Autodesk Inventor part; units mm, degrees
ref_plane "YZ Plane" through (0, 0, 0) normal (1, 0, 0) x (0, 1, 0)
ref_plane "XZ Plane" through (0, 0, 0) normal (0, 1, 0) x (-1, 0, 0)
ref_plane "XY Plane" through (0, 0, 0) normal (0, 0, 1) x (1, 0, 0)
sketch "Sketch1" plane through (0, 0, 0) normal (0, 1, 0) x (-1, 0, 0)
  circle A0 centre (0, 0) radius 17.5
  dimension "d0" = 35
extrude "Base" add sketch "Sketch1" along normal blind 10
sketch "Sketch2" plane through (0, 10, 0) normal (0, 1, 0) x (1, 0, 0)
  circle A0 centre (0, 0) radius 8
  circle A1 centre (-8, 0) radius 0.8
  dimension "d3" = 16
  dimension "d4" = 1.6
extrude "Mounting Hole" cut sketch "Sketch2" against normal through all contours A1 A0 | A0 A1 picked at (-7.7304, 0) picked at (-8.2616, 0.0332)
pattern_circular "Circular Pattern1" count 8 over 360 about axis through (0, 0, 0) along (0, 1, 0) of "Mounting Hole"
sketch "Sketch3" plane through (0, 10, 0) normal (0, 1, 0) x (1, 0, 0)
  arc A0 (-16.6435, 5.4078) -> (-17.5, 0) centre (0, 0) ccw
  line L0 (0, 0) -> (-16.6435, 5.4078) construction
  line L1 (0, 0) -> (-17.5, 0) construction
  line L2 (0, 0) -> (-25.2614, 4.001)
  line L3 (0, 0) -> (25.5763, 0) construction
  line L4 (-17.5, 0) -> (-21.2042, 3.3584)
  line L5 (-16.6435, 5.4078) -> (-21.2042, 3.3584)
  dimension "d11" = 18
  dimension "d12" = 171
  dimension "d13" = 5
extrude "Gear Tooth" add sketch "Sketch3" against normal blind 10
pattern_circular "Circular Pattern2" count 20 over 360 about axis through (0, 0, 0) along (0, 1, 0) of "Gear Tooth"
sketch "Sketch6" plane through (0, 10, 0) normal (0, 1, 0) x (1, 0, 0)
  point P0 (0, 0)
sketch "Sketch7" plane through (0, 10, 0) normal (0, 1, 0) x (1, 0, 0)
  circle A0 centre (0, 0) radius 10
  dimension "d26" = 20
extrude "Extrusion6" cut sketch "Sketch7" against normal blind 2
sketch "Sketch8" plane through (0, 8, 0) normal (0, 1, 0) x (1, 0, 0)
  circle A0 centre (0, 0) radius 4
  dimension "d29" = 8
extrude "Extrusion7" cut sketch "Sketch8" against normal blind 1.9
sketch "Sketch9" plane through (0, 6.1, 0) normal (0, 1, 0) x (1, 0, 0)
  circle A0 centre (0, 0) radius 2.25
  dimension "d32" = 4.5
extrude "Extrusion8" cut sketch "Sketch9" against normal blind 2.5
properties part number "JointSmallGear"
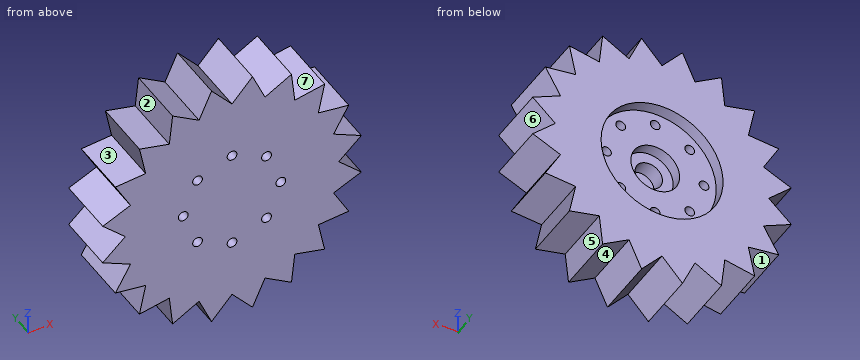
Here's how the part is built. I have some questions about the finished solid (model axes, mm). Face numbers are marked on the shaded views. A direction names the side the tool comes from. Give positions to 0.01 mm unless a question says otherwise; leave off trailing zeros. Loops run counter-clockwise (first coordinate to the right, second up) from the corner with the lowest first, then second, coordinate; pieces in that order, holes last. Notation, with made-up numbers: (45, -11.75) -> (62, -11.75) arc R14 cw to (62, 5.25) -> close; hole circle Ø10 at (4, 74.5). An arc over 180 degrees is marked (long way). Use one line per item in the form item = value. Start each with the question number.
1) Thinking about a two-plate mould opening in Z: for the marked faces 1, 2, 3 and 4, which applies, +Z half, -Z half, draft (parallel to the pull), parting line (faces both ways), or undercut?
2) Imagine slicing it at A-A (x = -8). Please give me the cut outline in (y, z), then the cut area to 3 significant figures.
3) Which directions (+Z, -Z, +X, -X, +Y, -Y) give clear straight access to the entire face, cutting with the end or side of a thin tool? Please do the marked faces 5, 6 and 7.
4) Imagine slicing it at C-C (y = 5.25). Count the separate pieces of the cut face and the enclosed holes in it, then the cut area to 3 significant figures.
5) Please list where these lines run through material, in increasing order: line 1 along X through (y, z) = (7.5, -17); line 2 along X through (y, z) = (5.75, -6); line 3 along Z through (x, y) = (5, 1.5).
6) For P1, Ø3, axis at y = 7, z = 7.5, coming from the -X side; P2, Ø1.8, axis at x = 0, z = -8, coming from the -Y side; P3, Ø1.8, axis at x = 5.66, z = -5.66, coming from the +Y side; P4, Ø6, axis at x = 0, z = 0, coming from the +Y side, each with a flat end and sliding along its axis, tell me the tip position at first contact or that it passes through.
7) Imagine slicing it at B-B (z = 8). Please give me the cut outline in (x, y).
Check values:
q1.face_1 = undercut
q1.face_2 = +Z half
q1.face_3 = undercut
q1.face_4 = -Z half
q2.outline = (0, -18.13) -> (10, -18.13) -> (10, -6) -> (8, -6) -> (8, -0.8) -> (0, -0.8) -> close; (0, 0.8) -> (8, 0.8) -> (8, 6) -> (10, 6) -> (10, 18.13) -> (0, 18.13) -> close
q2.area = 326 mm^2
q3.face_5 = -Z, +Y, -Y
q3.face_6 = +X, +Y, -Y
q3.face_7 = +Z, +Y, -Y
q4.separate_pieces = 1
q4.enclosed_holes = 9
q4.area = 1,140 mm^2
q5.line_1 = -9.98 to -6.03, -5.25 to 5.25, 6.03 to 9.98
q5.line_2 = -16.98 to -6.38, -4.93 to 4.93, 6.38 to 16.98
q5.line_3 = -17.55 to -6.11, -5.2 to 5.2, 6.11 to 17.55
q6.P1 = -18.7
q6.P2 = 0
q6.P3 = 8
q6.P4 = 6.1
q7.outline = (-18.13, 0) -> (-0.8, 0) -> (-0.8, 8) -> (-6, 8) -> (-6, 10) -> (-18.13, 10) -> close; (0.8, 0) -> (18.13, 0) -> (18.13, 10) -> (6, 10) -> (6, 8) -> (0.8, 8) -> close
